Part model, mm, in its own coordinate system. Round coordinates to 2 decimals unless told otherwise and drop trailing zeros. Loops run counter-clockwise (first coordinate to the right, second up) from the corner with the lowest first, then second, coordinate; pieces in that order, holes last. Notation, with made-up numbers: M 31,20.25 L 36,20.25 A32 cw 36,46.25 Z; hole C 13,12 d1. An arc over 180 degrees is marked long. Write each question's results on one line, items separated by ' | '.
from build123d import *

# Parameters (mm, degrees)
BOSS_EXTRUDE1_DEPTH = 5
SKETCH2_R           = 2
CUT_EXTRUDE1_DEPTH  = 10


with BuildPart() as part:
    # Sketch1 → Boss-Extrude1 (new body)
    with BuildSketch(Plane(origin=(0, 0, 0), x_dir=(1, 0, 0), z_dir=(0, 1, 0))):
        with BuildLine():
            Line((34, -89), (33, -89))
            ThreePointArc((33, -89), (32.292893219, -89.292893219), (32, -90))
            Line((32, -90), (32, -95))
            ThreePointArc((32, -95), (31.707106781, -95.707106781), (31, -96))
            Line((31, -96), (23, -96))
            ThreePointArc((23, -96), (22.292893219, -95.707106781), (22, -95))
            Line((22, -95), (22, -90))
            ThreePointArc((22, -90), (21.707106781, -89.292893219), (21, -89))
            Line((21, -89), (-21, -89))
            ThreePointArc((-21, -89), (-21.707106781, -89.292893219), (-22, -90))
            Line((-22, -90), (-22, -95))
            ThreePointArc((-22, -95), (-22.292893219, -95.707106781), (-23, -96))
            Line((-23, -96), (-31, -96))
            ThreePointArc((-31, -96), (-31.707106781, -95.707106781), (-32, -95))
            Line((-32, -95), (-32, -90))
            ThreePointArc((-32, -90), (-32.292893219, -89.292893219), (-33, -89))
            Line((-33, -89), (-34, -89))
            ThreePointArc((-34, -89), (-34.707106781, -88.707106781), (-35, -88))
            Line((-35, -88), (-35, 88))
            ThreePointArc((-35, 88), (-34.707106781, 88.707106781), (-34, 89))
            Line((-34, 89), (-33, 89))
            ThreePointArc((-33, 89), (-32.292893219, 89.292893219), (-32, 90))
            Line((-32, 90), (-32, 95))
            ThreePointArc((-32, 95), (-31.707106781, 95.707106781), (-31, 96))
            Line((-31, 96), (-23, 96))
            ThreePointArc((-23, 96), (-22.292893219, 95.707106781), (-22, 95))
            Line((-22, 95), (-22, 90))
            ThreePointArc((-22, 90), (-21.707106781, 89.292893219), (-21, 89))
            Line((-21, 89), (21, 89))
            ThreePointArc((21, 89), (21.707106781, 89.292893219), (22, 90))
            Line((22, 90), (22, 95))
            ThreePointArc((22, 95), (22.292893219, 95.707106781), (23, 96))
            Line((23, 96), (31, 96))
            ThreePointArc((31, 96), (31.707106781, 95.707106781), (32, 95))
            Line((32, 95), (32, 90))
            ThreePointArc((32, 90), (32.292893219, 89.292893219), (33, 89))
            Line((33, 89), (34, 89))
            ThreePointArc((34, 89), (34.707106781, 88.707106781), (35, 88))
            Line((35, 88), (35, -88))
            ThreePointArc((35, -88), (34.707106781, -88.707106781), (34, -89))
        make_face()
    extrude(amount=BOSS_EXTRUDE1_DEPTH)

    # Sketch2 → Cut-Extrude1 (cut)
    with BuildSketch(Plane(origin=(0, 5, 0), x_dir=(1, 0, 0), z_dir=(0, 1, 0))):
        with Locations((0, 73)):
            Circle(SKETCH2_R)
        with Locations((0, 53.061)):
            Circle(SKETCH2_R)
        with Locations((0, 11.061)):
            Circle(SKETCH2_R)
        with Locations((0, 31)):
            Circle(SKETCH2_R)
        with Locations((0, -30.939)):
            Circle(SKETCH2_R)
        with Locations((0, -11)):
            Circle(SKETCH2_R)
        with Locations((0, -72.939)):
            Circle(SKETCH2_R)
        with Locations((0, -53)):
            Circle(SKETCH2_R)
    extrude(amount=-CUT_EXTRUDE1_DEPTH, mode=Mode.SUBTRACT)


solid = part.part
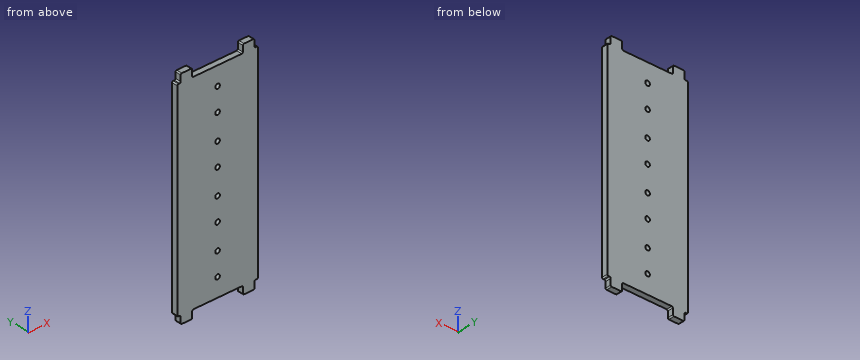
Item 1: Band-saw the part on A-A on z = 53. Give the cut face in (x, y), and give its area (3 significant figures).
Filled sheet:
outline: M -35,0 L -2,0 L -2,5 L -35,5 Z; M 2,0 L 35,0 L 35,5 L 2,5 Z | area: 330 mm^2
Item 2: Wall check: L1, parallel to X at y = 1.85, z = 11; L2, parallel to Z at x = 14.5, y = 0.95; L3, parallel to X at y = 0.65, z = 11.5. Give the ranges that are in metal, low to high.
Filled sheet:
L1: -35 to -2, 2 to 35 | L2: -89 to 89 | L3: -35 to -1.94, 1.94 to 35
Item 3: Drop flat-ended pins along their axis: P1, Ø10, axis at x = -18, z = 15, coming from the -Y side; P2, Ø2.5, axis at x = 0, z = -53.061, coming from the -Y side; P3, Ø1.5, axis at y = 3.5, z = -93.5, coming from the -X side; P4, Ø1.1, axis at x = -33.5, y = 2, coming from the -Z side. Give the stop position or say it passes through.
Filled sheet:
P1: y = 0 | P2: through | P3: x = -32 | P4: z = -89
Item 4: Band-saw the part on B-B on x = 0. Count the separate pieces of the cut face and the enclosed holes in it, and give its area (3 significant figures).
Filled sheet:
separate pieces: 9 | enclosed holes: 0 | area: 730 mm^2
Item 5: Band-saw the part on C-C on x = -16. Give the cut face in (y, z).
Filled sheet:
outline: M 0,-89 L 5,-89 L 5,89 L 0,89 Z
